```python
from build123d import *

# Parameters (mm, degrees)
F1_DEPTH = 63.5
F0_W     = 24.1857025899
F0_H     = 19.05
F2_DEPTH = 25.4
F3_DEPTH = 7.9375
F5_R     = 6.35


with BuildPart() as f1:
    # F0 (on Front) → F1 (new body, symmetric)
    with BuildSketch(Plane.XZ):
        Polygon((22.225, 9.525), (-41.275, 9.525), (-41.275, -9.525), (41.275, -9.525), (41.275, 9.525), align=None)
    extrude(amount=F1_DEPTH, both=True)

    # F0 (on Front) → F2 (join, symmetric)
    with BuildSketch(Plane.XZ):
        with BuildLine():
            Line((22.225, 27.0002), (22.225, 9.525))
            Line((22.225, 9.525), (41.275, 9.525))
            Line((41.275, 9.525), (41.275, 27.0002))
            ThreePointArc((41.275, 27.0002), (45.9246798487, 38.2255201513), (57.15, 42.8752))
            Line((57.15, 42.8752), (57.15, 61.9252))
            add(Edge.make_bspline(
                [(54.2900015648, 61.8079007852), (55.2509849967, 61.8452258423), (56.2046080591, 61.8840829618), (57.15, 61.9252)],
                knots=[108.9404327858, 108.9404327858, 108.9404327858, 108.9404327858, 111.5045361635, 111.5045361635, 111.5045361635, 111.5045361635], degree=3))
            ThreePointArc((54.2900015648, 61.8079007852), (31.4630279096, 50.6631476149), (22.225, 27.0002))
        make_face()
        with Locations((69.2428512949, 52.4002)):
            Rectangle(F0_W, F0_H)
    extrude(amount=F2_DEPTH, both=True)

    # F0 (on Front) → F3 (join, symmetric)
    with BuildSketch(Plane.XZ):
        with BuildLine():
            add(Edge.make_bspline(
                [(-41.275, 9.525), (-40.6545165411, 61.4018227943), (13.4609336457, 60.2220802175), (54.2900015648, 61.8079007852)],
                knots=[0, 0, 0, 0, 108.9404327858, 108.9404327858, 108.9404327858, 108.9404327858], degree=3))
            Line((-41.275, 9.525), (22.225, 9.525))
            Line((22.225, 9.525), (22.225, 27.0002))
            ThreePointArc((22.225, 27.0002), (31.4630279096, 50.6631476149), (54.2900015648, 61.8079007852))
        make_face()
    extrude(amount=F3_DEPTH, both=True)

    # F0 (on Front) → F4 (revolve)
    with BuildSketch(Plane.XZ):
        Polygon((81.3357025899, 66.675), (81.3357025899, 61.9252), (81.3357025899, 42.8752), (81.3357025899, 38.1), (107.95, 38.1), (107.95, 66.675), align=None)
    revolve(axis=Axis((81.3357025899, 0, 52.3875), (0, 0, 1)))

    # F5
    f5_edges = [f1.edges().sort_by_distance(p)[0] for p in [
        (41.275, -63.5, 0),
        (-41.275, -63.5, 0),
        (41.275, 63.5, 0),
        (-41.275, 63.5, 0),
    ]]
    fillet(f5_edges, radius=F5_R)


solid = f1.part
```
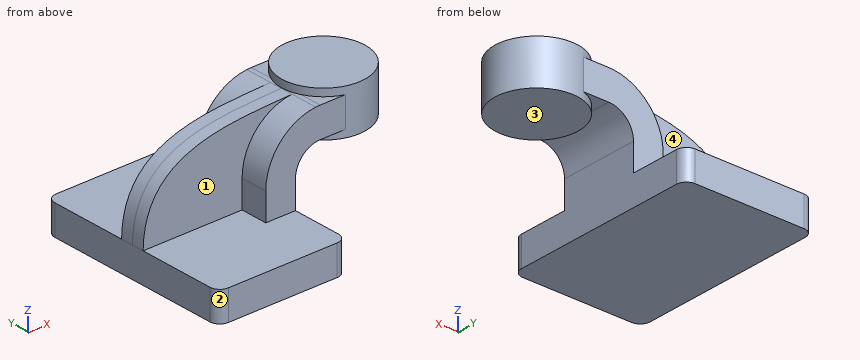
Geometry: final body of the model. Coordinates: model frame, mm. Face numbers are marked on the shaded views. A direction names the side the tool comes from. Coordinates: 2 decimals unless noted, no trailing zeros. Order: outer loops, then holes, each group sorted by start corner. A loop starts at its lowest first (then second) coordinate and runs counter-clockwise, first axis right, second up. Notation, with made-up numbers: M 83,85.5 L 119,85.5 A26 cw 119,123.5 Z; hole C -40,-19.75 d9. An arc over 180 degrees is marked long. Answer as CSV lines item,"result".
Q1. Line query: probe 1 along Y at (x, z) = (60, 52.5); probe 2 along Y at (x, z) = (-23, 37); probe 3 along Z at (x, y) = (27, 28.5) (3 decimals). Output: solid intervals per line, ascending. Write a range as [from, to].
Answers:
probe 1,"y = [-25.4, 25.4]"
probe 2,"y = [-7.94, 7.94]"
probe 3,"z = [-9.525, 9.525]"
Q2. Section B-B on y = -48.5. Return the cut outline in (x, z) (3 decimals).
Answers:
outline,"M -41.275,-9.525 L 41.275,-9.525 L 41.275,9.525 L -41.275,9.525 Z"
Q3. Set-up query: the marked faces 1, 2, 3 and 4. Return all of +Z, -Z, +X, -X, +Y, -Y with unobstructed straight access to the full face (end or side cutting, diameter ignored); none if empty.
Answers:
face 1,"+Z, -X, -Y"
face 2,"+Z, -Z, -X, -Y"
face 3,"-Z, +X, +Y, -Y"
face 4,"+Z, -X, +Y"
Q4. First-contact query: P1, Ø5, axis at y = 28, z = 11, coming from the -X side (3 decimals); P2, Ø3, axis at y = -20, z = 17, coming from the -X side (3 decimals); P3, Ø3, axis at x = 57, y = 21.5, coming from the +Z side; P4, Ø8, axis at x = 53, y = 3.5, coming from the -Z side. Flat tips, straight axial feed; report the tip coordinate or a pass-through.
Answers:
P1,"stops at x = -41.275"
P2,"stops at x = 22.225"
P3,"stops at z = 61.93"
P4,"stops at z = 38.1"
Q5. Section A-A on z = 3. Return the cut outline in (x, y) (3 decimals).
Answers:
outline,"M -41.275,-57.15 A6.35 ccw -34.925,-63.5 L 34.925,-63.5 A6.35 ccw 41.275,-57.15 L 41.275,57.15 A6.35 ccw 34.925,63.5 L -34.925,63.5 A6.35 ccw -41.275,57.15 Z"
Q6. Section C-C on x = 87. Return the cut outline in (y, z) (3 decimals), and give its area (3 significant figures).
Answers:
outline,"M -26.005,38.1 L 26.005,38.1 L 26.005,66.675 L -26.005,66.675 Z"
area,"1,490 mm^2"
